Here's how the part is built. I have some questions about the finished solid (model axes, mm). A direction names the side the tool comes from. Round coordinates to 2 decimals unless told otherwise and drop trailing zeros. Write each loop counter-clockwise with the first axis right and the second up, starting at its lowest first coordinate (ties: lowest second). Pieces come first, ordered by that corner, then holes. Notation, with made-up numbers: M 65,28.25 L 79,28.25 A15 ccw 79,56.25 Z; hole C -32,71.5 d9. An arc over 180 degrees is marked long. Use a Markdown table: item, result. Add a question column.
```python
from build123d import *

# Parameters (mm, degrees)
SKETCH1_W               = 98
SKETCH1_H               = 111.829224908
SKETCH1_R               = 0.85
SKETCH1_W_2             = 23.8
SKETCH1_H_2             = 14.4
BOSS_EXTRUDE1_DEPTH     = 5
SKETCH3_W               = 98
SKETCH3_H               = 3
BOSS_EXTRUDE2_DEPTH     = 70
SKETCH4_W               = 61
SKETCH4_H               = 5.5
CUT_EXTRUDE1_DEPTH      = 50
CUT_EXTRUDE2_DEPTH      = 103.114856343
CUT_EXTRUDE2_DEPTH_BACK = 103.114856343
SKETCH5_W               = 98
SKETCH5_H               = 45.714612454
SKETCH6_W               = 8
SKETCH6_H               = 60
BOSS_EXTRUDE3_DEPTH     = 15
CUT_EXTRUDE3_DEPTH      = 109.037687776
BOSS_EXTRUDE4_DEPTH     = 6.114612454


with BuildPart() as part:
    # Sketch1 → Boss-Extrude1 (new body)
    with BuildSketch(Plane.XY):
        Rectangle(SKETCH1_W, SKETCH1_H)
        with Locations((14, 0)):
            Circle(SKETCH1_R, mode=Mode.SUBTRACT)
        with Locations((-14, 0)):
            Circle(SKETCH1_R, mode=Mode.SUBTRACT)
        Rectangle(SKETCH1_W_2, SKETCH1_H_2, mode=Mode.SUBTRACT)
    extrude(amount=BOSS_EXTRUDE1_DEPTH)

    # Sketch3 → Boss-Extrude2 (add)
    with BuildSketch(Plane(origin=(0, 0, 0), x_dir=(-1, 0, 0), z_dir=(0, 0, -1))):
        with Locations((0, -8.7)):
            Rectangle(SKETCH3_W, SKETCH3_H)
    extrude(amount=BOSS_EXTRUDE2_DEPTH)

    # Sketch4 → Cut-Extrude1 (cut)
    with BuildSketch(Plane(origin=(0, -7.2, 0), x_dir=(1, 0, 0), z_dir=(0, 1, 0))):
        with Locations((0, 35.75)):
            Rectangle(SKETCH4_W, SKETCH4_H)
    extrude(amount=-CUT_EXTRUDE1_DEPTH, mode=Mode.SUBTRACT)

    # Sketch5 → Cut-Extrude2 (cut, two sides: drawn at the far end of the back side and taken through both)
    with BuildSketch(Plane(origin=(0, 0, 0), x_dir=(-1, 0, 0), z_dir=(0, 0, -1)).offset(-CUT_EXTRUDE2_DEPTH_BACK)):
        with Locations((0, -33.057306227)):
            Rectangle(SKETCH5_W, SKETCH5_H)
    extrude(amount=CUT_EXTRUDE2_DEPTH + CUT_EXTRUDE2_DEPTH_BACK, mode=Mode.SUBTRACT)

    # Sketch6 → Boss-Extrude3 (add)
    with BuildSketch(Plane.XY.offset(5)):
        with Locations((22.52, 25.914612454)):
            Rectangle(SKETCH6_W, SKETCH6_H)
    extrude(amount=BOSS_EXTRUDE3_DEPTH)

    # Sketch7 → Cut-Extrude3 (cut, through all)
    with BuildSketch(Plane(origin=(0, 55.914612454, 0), x_dir=(1, 0, 0), z_dir=(0, 1, 0))):
        Polygon((18.52, -9.1), (21.92, -9.1), (21.92, -7.1), (24.32, -7.1), (24.32, -18.5), (21.92, -18.5), (21.92, -16.5), (18.52, -16.5), align=None)
    extrude(amount=-CUT_EXTRUDE3_DEPTH, mode=Mode.SUBTRACT)

    # Sketch8 → Boss-Extrude4 (add)
    with BuildSketch(Plane.XZ.offset(4.085387546)):
        Polygon((21.92, 7.1), (21.92, 9.1), (18.52, 9.1), (18.52, 5), (26.52, 5), (26.52, 20), (18.52, 20), (18.52, 16.5), (21.92, 16.5), (21.92, 18.5), (24.32, 18.5), (24.32, 7.1), align=None)
    extrude(amount=BOSS_EXTRUDE4_DEPTH)


solid = part.part
```
Item 1: Imagine slicing it at A-A on z = 2. List the corners of the cut face in (x, y) for me.
Item 2: For pin 1 Ø1.6 at (y, z) = (36.5, 17.5) entering from +X; pin 2 Ø2 at (x, y) = (-31.5, 19) entering from -Z; pin 3 Ø8 at (x, y) = (36.5, 26) entering from +Z; pin 4 Ø1.4 at (x, y) = (14, 0) entering from -Z, each with a flat end and sliding along its axis, tell me the tip position at first contact or that it passes through.
Item 3: Imagine slicing it at C-C on x = 32.5. List the corners of the cut face in (y, z) for me.
Item 4: I need wall thicknesses on probe 1 along Z at (x, y) = (22.5, 51); probe 2 along Y at (x, z) = (-14, 3.95); probe 3 along X at (y, z) = (19, 12). Which ranges of each line are inside material? Lowest first, please. Write a range as from..to.
Item 5: Imagine slicing it at D-D on y = 38. List the corners of the cut face in (x, z) for me.
Item 6: If we mould it in two halves opening along Z, with no side actions, what happens to faces 6 (the face through (23, 23, 18.5)), 7 (the face through (3, 55.915, 3)), 8 (the face through (23, 23, 20))? For each: +Z half, -Z half, draft (parallel to the pull), parting line (faces both ways), or undercut.
Item 7: On a 3-axis mill with a long thin cutter (end or side, diameter ignored), from which of +Z, -Z, +X, -X, +Y, -Y can I reach the whole of each face in a straight line? I mean faces 1 (the face through (20, 23, 9.1)), 2 (the face through (-1, 25, 0)), 3 (the face through (-11.9, 0, 2)), 4 (the face through (18.52, 23, 7)), 5 (the face through (23, 23, 7.1)). Say none if no direction works.
Item 8: Imagine slicing it at B-B on x = -27.5. List the corners of the cut face in (y, z) for me, plus the area to 3 significant figures.
The answers:
| question | item | result |
|---|---|---|
| 1 | outline | M -49,-10.2 L 49,-10.2 L 49,55.91 L -49,55.91 Z; hole C -14,0 d1.7; hole M -11.9,-7.2 L 11.9,-7.2 L 11.9,7.2 L -11.9,7.2 Z; hole C 14,0 d1.7 |
| 2 | pin 1 | x = 26.52 |
| 2 | pin 2 | z = 0 |
| 2 | pin 3 | z = 5 |
| 2 | pin 4 | through |
| 3 | outline | M -10.2,-70 L -7.2,-70 L -7.2,0 L 55.91,0 L 55.91,5 L -10.2,5 Z |
| 4 | probe 1 | 0..7.1, 18.5..20 |
| 4 | probe 2 | -10.2..-0.85, 0.85..55.91 |
| 4 | probe 3 | 24.32..26.52 |
| 5 | outline | M -49,0 L 49,0 L 49,5 L 26.52,5 L 26.52,20 L 18.52,20 L 18.52,16.5 L 21.92,16.5 L 21.92,18.5 L 24.32,18.5 L 24.32,7.1 L 21.92,7.1 L 21.92,9.1 L 18.52,9.1 L 18.52,5 L -49,5 Z |
| 6 | face 6 | undercut |
| 6 | face 7 | draft |
| 6 | face 8 | +Z half |
| 7 | face 1 | -X, +Y, -Y |
| 7 | face 2 | -Z, +X, -X, +Y |
| 7 | face 3 | +Z, -Z |
| 7 | face 4 | +Z, -X, +Y, -Y |
| 7 | face 5 | +Y, -Y |
| 8 | outline | M -10.2,-70 L -7.2,-70 L -7.2,-38.5 L -10.2,-38.5 Z; M -10.2,-33 L -7.2,-33 L -7.2,0 L 55.91,0 L 55.91,5 L -10.2,5 Z |
| 8 | area | 524 mm² |
